For this review, take the finished solid that the model builds, in its own axes (mm). Round coordinates to 2 decimals unless told otherwise and drop trailing zeros. Order: outer loops, then holes, each group sorted by start corner. A loop starts at its lowest first (then second) coordinate and runs counter-clockwise, first axis right, second up. Notation, with made-up numbers: (28, -7.5) - (56, -7.5) arc R30 ccw to (56, 19.5) - close; hole circle Ø6 at (-27.75, 11.5). An arc over 180 degrees is marked (long way). One line per question, with ' | ' between items.
Autodesk Inventor part; units mm, degrees
ref_plane "YZ Plane" through (0, 0, 0) normal (1, 0, 0) x (0, 1, 0)
ref_plane "XZ Plane" through (0, 0, 0) normal (0, 1, 0) x (-1, 0, 0)
ref_plane "XY Plane" through (0, 0, 0) normal (0, 0, 1) x (1, 0, 0)
sketch "Sketch1" plane through (0, 0, 0) normal (0, 0, 1) x (1, 0, 0)
  line L0 (0, 0) -> (293.4944, 0) construction
  line L1 (293.4944, 0) -> (293.4944, -132.0217) construction
  line L2 (293.4944, -132.0217) -> (0, -132.0217) construction
  line L3 (0, -132.0217) -> (0, 0) construction
  line L4 (79.3681, -56.3049) -> (159.3681, -56.3049) construction
  line L5 (283.1562, -93.1287) -> (274.2161, -88.6482) construction
  line L6 (283.1562, -93.1287) -> (282.3201, -93.1287) construction
  line L7 (18.3483, -97.5091) -> (27.4302, -93.3236) construction
  line L8 (18.3483, -97.5091) -> (20.5956, -97.5091) construction
  arc A0 (103.0994, -81.9859) -> (27.4302, -93.3236) centre (93.4367, -275.677) ccw
  arc A1 (274.2161, -88.6482) -> (204.4098, -79.893) centre (217.7822, -255.937) ccw
  arc A2 (103.0994, -81.9859) -> (204.4098, -79.893) centre (140.8276, 544.7964) ccw
  line L9 (27.4302, -93.3236) -> (27.4302, -72.2735)
  line L10 (27.4302, -72.2735) -> (272.6166, -67.591)
  line L11 (272.6166, -67.591) -> (274.2161, -88.6482)
  line L12 (103.0994, -81.9859) -> (86.3195, -71.1488) construction
  line L13 (204.4098, -79.893) -> (220.9707, -68.5773) construction
  line L14 (86.3195, -71.1488) -> (86.3195, -81.1488) construction
  line L15 (86.3195, -81.1488) -> (103.0994, -81.9859) construction
  line L16 (220.9707, -68.5773) -> (221.7303, -78.5773) construction
  line L17 (221.7303, -78.5773) -> (204.4098, -79.893) construction
  dimension "d5" = 80
  dimension "d85" = 10
  dimension "d87" = 26.619
  dimension "d92" = 10
  dimension "d94" = 24.743
  dimension "d100" = 22.985
  dimension "d101" = 22.755
  dimension "d106" = 10
  dimension "d111" = 10
  dimension "d112" = 30
  dimension "d113" = 30
extrude "Extrusion1" add sketch "Sketch1" along normal blind 10
sketch "Sketch2" plane through (0, 0, 10) normal (0, 0, 1) x (1, 0, 0)
  arc A0 (103.0994, -81.9859) -> (204.4098, -79.893) centre (140.8276, 544.7964) ccw
  line L0 (272.6166, -67.591) -> (27.4302, -72.2735)
  line L1 (27.4302, -72.2735) -> (27.4302, -93.3236)
  line L2 (274.2161, -88.6482) -> (272.6166, -67.591)
  line L3 (125.3768, -83.1204) -> (158.7723, -83.1204)
  line L4 (140.8276, -83.1204) -> (140.8276, -70.1078)
  line L5 (140.8276, -76.6141) -> (27.4302, -76.6141)
  line L6 (140.8276, -76.6141) -> (273.302, -76.6141)
  arc A1 (274.2161, -88.6482) -> (204.4098, -79.893) centre (217.7822, -255.937) ccw
  line L7 (274.2161, -88.6482) -> (272.6166, -67.591)
  line L8 (272.6166, -67.591) -> (27.4302, -72.2735)
  line L9 (27.4302, -72.2735) -> (27.4302, -93.3236)
  arc A2 (103.0994, -81.9859) -> (27.4302, -93.3236) centre (93.4367, -275.677) ccw
  arc A3 (103.0994, -81.9859) -> (204.4098, -79.893) centre (140.8276, 544.7964) ccw
  line L10 (140.8276, -83.1204) -> (140.4575, -63.7401)
  point P0 (0, 0)
  point P1 (204.4098, -79.893)
  point P2 (140.5792, -70.1126)
  point P3 (140.7034, -76.6141)
  dimension "d121" = 113.3974
  dimension "d122" = 132.4743
extrude "Extrusion2" cut sketch "Sketch2" against normal blind 10 contours L4 L6 L2 A1 A0 | L10 L5 L4 | L5 L10 L0 L4 | L4 L0 L2 L6
sketch "Sketch4" plane through (0, 0, 10) normal (0, 0, 1) x (1, 0, 0)
  line L0 (140.5792, -70.1126) -> (27.4302, -72.2735)
  line L1 (27.4302, -72.2735) -> (27.4302, -93.3236)
  arc A0 (103.0994, -81.9859) -> (27.4302, -93.3236) centre (93.4367, -275.677) ccw
  arc A1 (103.0994, -81.9859) -> (140.8276, -83.1204) centre (140.8276, 544.7964) ccw
  line L2 (27.4302, -72.2735) -> (27.4302, -93.3236)
  arc A2 (103.0994, -81.9859) -> (27.4302, -93.3236) centre (93.4367, -275.677) ccw
  line L3 (27.4302, -72.2735) -> (27.8295, -93.1796)
  line L4 (140.8276, -83.1204) -> (140.5792, -70.1126)
  point P0 (0, 0)
  point P1 (253.7282, -67.9517)
  dimension "d128" = 90
extrude "Extrusion4" cut sketch "Sketch4" against normal blind 10 contours L3 A0 L1
equation "\"d111\" = d106"
equation "\"d113\" = d112"
properties part number "deseczka_dol_check"
(1) We need section C-C on y = -91.25. State the section outline as (x, z) points.
Output values:
outline: (27.79, 0) - (33.47, 0) - (33.47, 10) - (27.79, 10) - close
(2) For probe 1 along Y at (x, z) = (72.5, 4); probe 2 along Y at (x, z) = (91, 4.25); probe 3 along X at (y, z) = (-75.25, 4), list the stretches that pass through material, from the lowest coordinate up. Write a range as [from, to].
Output values:
probe 1: [-82.88, -71.41] | probe 2: [-81.76, -71.06] | probe 3: [27.49, 140.68]
(3) Insertion check: pin 1 (2 mm diameter, centred on y = -88.5, z = 5, fed in from -X); pin 2 (4 mm diameter, centred on y = -85.5, z = 8.5, fed in from -X); pin 3 (5 mm diameter, centred on x = 98.5, y = -86.5, fed in from -Z); pin 4 (1.5 mm diameter, centred on x = 125.5, z = 4, fed in from +Y). Each pin has a flat end and moves straight along its axis. Give the tip position at first contact, or say it passes through.
Output values:
pin 1: x = 27.72 | pin 2: x = 27.64 | pin 3: through | pin 4: y = -70.39
(4) Mouldability with a two-part tool opening along X and no side actions: class faces 1 (the flat face through (83, -79, 10)), 2 (the cylindrical face through (64.38, -83.934, 4.93)), 3 (the cylindrical face through (122.219, -82.845, 4.93)) as released by +X, released by -X, zero draft, split by the parting line, or undercut.
Output values:
face 1: zero draft | face 2: undercut | face 3: undercut
(5) We need section A-A on z = 5. State the section outline as (x, y) points, plus the area to 3 significant figures.
Output values:
outline: (27.43, -72.27) - (27.83, -93.18) arc R193.93 cw to (103.1, -81.99) arc R627.93 ccw to (140.83, -83.12) - (140.58, -70.11) - close | area: 1,480 mm^2
(6) We need section B-B on x = 58. State the section outline as (y, z) points, plus the area to 3 significant figures.
Output values:
outline: (-85.01, 0) - (-71.69, 0) - (-71.69, 10) - (-85.01, 10) - close | area: 133 mm^2
